Geometry check sheet. Reference: the model listing, model coordinates, mm. Round coordinates to 2 decimals unless told otherwise and drop trailing zeros. Order: outer loops, then holes, each group sorted by start corner. A loop starts at its lowest first (then second) coordinate and runs counter-clockwise, first axis right, second up. Notation, with made-up numbers: M -13.5,88 L -3.5,88 A19 ccw -3.5,103 Z; hole C 80,-19.75 d4. An arc over 180 degrees is marked long. Answer as a JSON object with one key per item and string values. Group by question number.
Autodesk Inventor part; units mm, degrees
ref_plane "YZ Plane" through (0, 0, 0) normal (1, 0, 0) x (0, 1, 0)
ref_plane "XZ Plane" through (0, 0, 0) normal (0, 1, 0) x (-1, 0, 0)
ref_plane "XY Plane" through (0, 0, 0) normal (0, 0, 1) x (1, 0, 0)
sketch "Sketch1" plane through (0, 0, 0) normal (0, 0, 1) x (1, 0, 0)
  line L0 (0, 0) -> (10, 0) construction
  line L1 (0, -4) -> (10, -4)
  line L2 (10, 4) -> (0, 4)
  arc A0 (0, 4) -> (0, -4) centre (0, 0) ccw
  arc A1 (10, -4) -> (10, 4) centre (10, 0) ccw
  point P0 (5, 0)
  dimension "d0" = 10
  dimension "d1" = 4
extrude "Extrusion1" add sketch "Sketch1" against normal blind 3
hole "Hole1" at (0, 0, 0) at (10, 0, 0) direction (0, 0, -1) diameter 3 depth 8 tip angle 118
properties part number "Updown_link"
1) Thickness scan on line 1 along X through (y, z) = (0, -1.15); line 2 along Y through (x, z) = (0, -1.8); line 3 along X through (y, z) = (-0.5, -1.15). Record the ranges inside material, lowest first. Write a range as [from, to].
2) Sectioned sample at D-D (y = -2.25). Record the boundary of the cut face in (x, z), then the cut area to 3 significant figures.
3) Sectioned sample at C-C (x = 0.75). Record the boundary of the cut face in (y, z), then the cut area to 3 significant figures.
4) Sectioned sample at B-B (z = -2.25). Record the boundary of the cut face in (x, y).
5) Release check for a two-part mould opening along X. For faces 1 (the cylindrical face through (14, 0, -1)), 2 (the cylindrical face through (-0.07, 1.5, -1.52)), 3 (the flat face through (5, 0, -3)), 4 (the cylindrical face through (11.464, 0.325, -1.521)) record: +X half, -X half, draft (parallel to the pull), parting line (faces both ways), or undercut.
6) Sectioned sample at A-A (y = 0). Record the boundary of the cut face in (x, z), then the cut area to 3 significant figures.
7) Go/stop test with flat-tipped pins: P1, Ø3, axis at x = 8.5, y = -2, coming from the +Z side; P2, Ø1.5, axis at x = 0, y = 0, coming from the -Z side. Record where each tip stops, or that it passes through.
Final values:
{
 "1": {"line 1": "x = [-4, -1.5], [1.5, 8.5], [11.5, 14]", "line 2": "y = [-4, -1.5], [1.5, 4]", "line 3": "x = [-3.97, -1.41], [1.41, 8.59], [11.41, 13.97]"},
 "2": {"outline": "M -3.31,-3 L 13.31,-3 L 13.31,0 L -3.31,0 Z", "area": "49.8 mm^2"},
 "3": {"outline": "M -4,-3 L -1.3,-3 L -1.3,0 L -4,0 Z; M 1.3,-3 L 4,-3 L 4,0 L 1.3,0 Z", "area": "16.2 mm^2"},
 "4": {"outline": "M 0,-4 L 10,-4 A4 ccw 10,4 L 0,4 A4 ccw Z; hole C 0,0 d3; hole C 10,0 d3"},
 "5": {"face 1": "+X half", "face 2": "undercut", "face 3": "draft", "face 4": "undercut"},
 "6": {"outline": "M -4,-3 L -1.5,-3 L -1.5,0 L -4,0 Z; M 1.5,-3 L 8.5,-3 L 8.5,0 L 1.5,0 Z; M 11.5,-3 L 14,-3 L 14,0 L 11.5,0 Z", "area": "36.0 mm^2"},
 "7": {"P1": "stops at z = 0", "P2": "passes through"}
}
